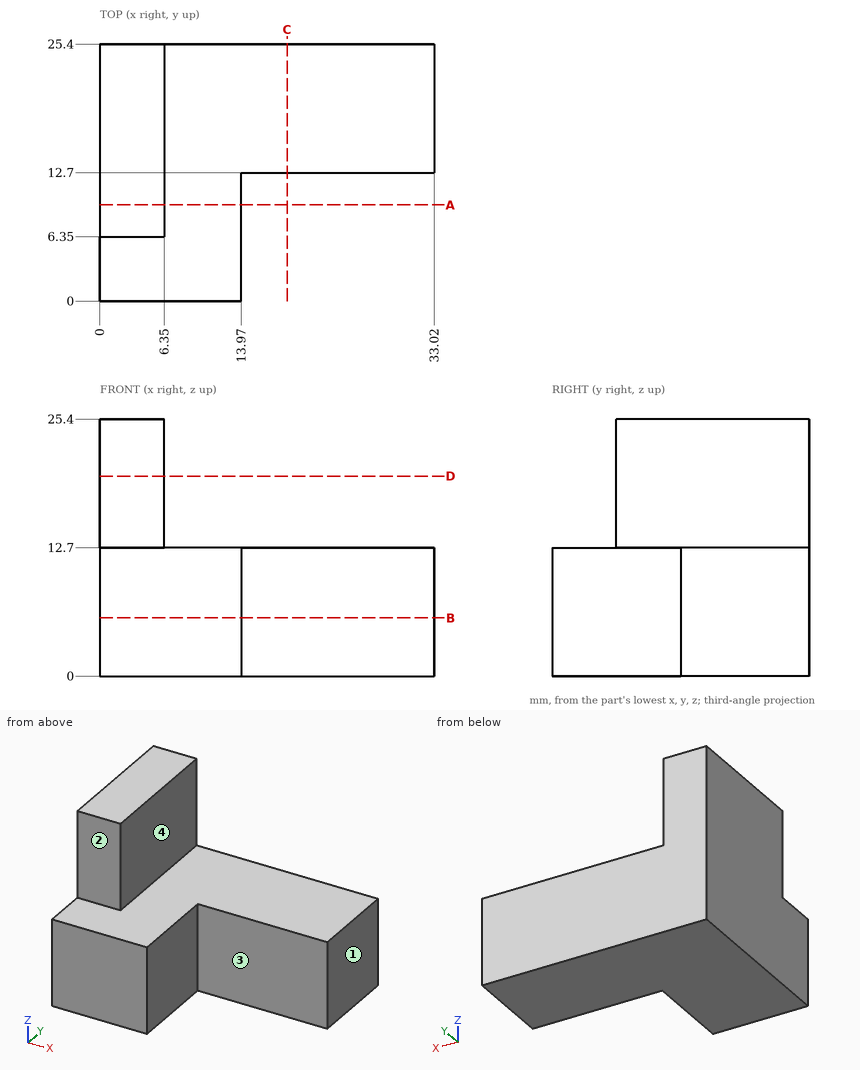
Source: three-view drawing plus pictorial views. Frame: mm from the lowest corner of the part. A direction names the side the tool comes from. Give positions to 0.01 mm unless a question says otherwise; leave off trailing zeros. Write each loop counter-clockwise with the first axis right and the second up, starting at its lowest first coordinate (ties: lowest second). Pieces come first, ordered by that corner, then holes. Notation, with made-up numbers: (59, 43.25) - (67, 43.25) arc R34 ccw to (67, 77.25) - close; hole circle Ø2 at (80, 0). An arc over 180 degrees is marked (long way). Write item = value, one per line. Start each with the question number.
Q1. Cut plane A-A, the plane y = 9.5. Return loops of the section in (x, z).
Q2. Material intervals for probe 1 along Z at (x, y) = (21.5, 21.75); probe 2 along Y at (x, z) = (30.5, 4.75); probe 3 along X at (y, z) = (2, 9.5), sorted ascending.
Q3. Cut plane C-C, the plane x = 18.5. Return loops of the section in (y, z), then the cut area to 3 significant figures.
Q4. Cut plane B-B, the plane z = 5.75. Return loops of the section in (x, y), then the cut area to 3 significant figures.
Q5. Pin query (flat end, axial travel): pin 1 Ø3 at (y, z) = (6, 15.5) entering from +X; pin 2 Ø5 at (x, y) = (6.5, 18) entering from +Z; pin 3 Ø6.5 at (y, z) = (3, 9) entering from +X; pin 4 Ø3 at (x, z) = (2.5, 19) entering from -Y. Return the tip coordinate at first contact, or that it passes through.
Q6. Cut plane D-D, the plane z = 19.75. Return loops of the section in (x, y), then the cut area to 3 significant figures.
Q7. Reachability of the marked faces 1, 2, 3 and 4 from +Z, -Z, +X, -X, +Y, -Y: full face, straight path, thin tool, end or side. Return the list, or none.
Computed values:
q1.outline = (0, 0) - (13.97, 0) - (13.97, 12.7) - (6.35, 12.7) - (6.35, 25.4) - (0, 25.4) - close
q2.probe_1 = 0 to 12.7
q2.probe_2 = 12.7 to 25.4
q2.probe_3 = 0 to 13.97
q3.outline = (12.7, 0) - (25.4, 0) - (25.4, 12.7) - (12.7, 12.7) - close
q3.area = 161 mm²
q4.outline = (0, 0) - (13.97, 0) - (13.97, 12.7) - (33.02, 12.7) - (33.02, 25.4) - (0, 25.4) - close
q4.area = 597 mm²
q5.pin_1 = 6.35
q5.pin_2 = 25.4
q5.pin_3 = 13.97
q5.pin_4 = 6.35
q6.outline = (0, 6.35) - (6.35, 6.35) - (6.35, 25.4) - (0, 25.4) - close
q6.area = 121 mm²
q7.face_1 = +Z, -Z, +X, +Y, -Y
q7.face_2 = +Z, +X, -X, -Y
q7.face_3 = +Z, -Z, +X, -Y
q7.face_4 = +Z, +X, +Y, -Y
